Geometry check sheet. Reference: the model listing, model coordinates, mm. Face numbers are marked on the shaded views. A direction names the side the tool comes from. Round coordinates to 2 decimals unless told otherwise and drop trailing zeros. Write each loop counter-clockwise with the first axis right and the second up, starting at its lowest first coordinate (ties: lowest second). Pieces come first, ordered by that corner, then holes. Notation, with made-up numbers: (-21.5, 37.25) - (32.5, 37.25) arc R19 cw to (32.5, 70.25) - close; hole circle Ø1 at (75.5, 42). An arc over 180 degrees is marked (long way). Return JSON: item names as keys, results as strings.
```python
from build123d import *

# Parameters (mm, degrees)
SALIENTE_EXTRUIR1_DEPTH = 10
CROQUIS2_R              = 1.5
CORTAR_EXTRUIR1_DEPTH   = 10


with BuildPart() as part:
    # Croquis1 → Saliente-Extruir1 (new body)
    with BuildSketch(Plane.XY):
        Polygon((0, 0), (53, 0), (53, 25), (51, 25), (51, 27), (53, 27), (53, 29), (51, 29), (51, 31), (55, 31), (55, -2), (-2, -2), (-2, 31), (2, 31), (2, 29), (0, 29), (0, 27), (2, 27), (2, 25), (0, 25), align=None)
    extrude(amount=SALIENTE_EXTRUIR1_DEPTH)

    # Croquis2 → Cortar-Extruir1 (cut)
    with BuildSketch(Plane.XZ.offset(2)):
        with Locations((45, 5)):
            Circle(CROQUIS2_R)
        with Locations((8, 5)):
            Circle(CROQUIS2_R)
    extrude(amount=-CORTAR_EXTRUIR1_DEPTH, mode=Mode.SUBTRACT)


solid = part.part
```
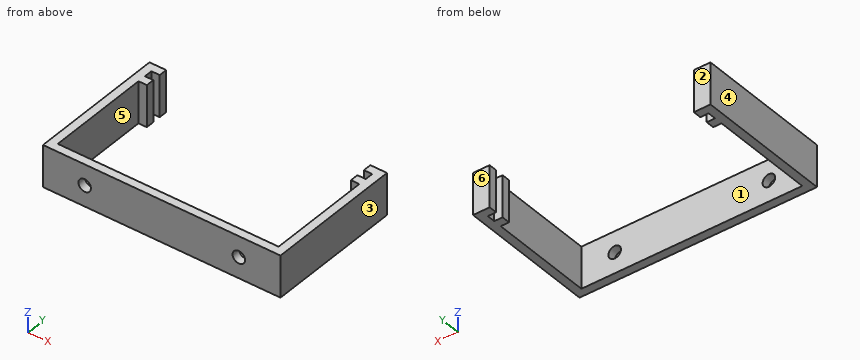
(1) Section check A-A, the plane x = 45. Enter the section's corners in (y, z), plus the area to 3 significant figures.
Response values:
{"outline": "(-2, 0) - (0, 0) - (0, 3.5) - (-2, 3.5) - close; (-2, 6.5) - (0, 6.5) - (0, 10) - (-2, 10) - close", "area": "14.0 mm^2"}
(2) Access from +Z, -Z, +X, -X, +Y, -Y to the whole of each face (thin tool, end or side, straight path). Record for the marked faces 5 and 6.
Response values:
{"face 5": "+Z, -Z", "face 6": "+Z, -Z, +X, -X, +Y"}
(3) Section check B-B, the plane y = 28. Enter the section's corners in (x, z), plus the area to 3 significant figures.
Response values:
{"outline": "(-2, 0) - (0, 0) - (0, 10) - (-2, 10) - close; (53, 0) - (55, 0) - (55, 10) - (53, 10) - close", "area": "40.0 mm^2"}
(4) Gauge pin test, flat end, axial feed: pin 1 (2 mm diameter, centred on x = 16, z = 3.5, fed in from +Y). Record the tip position at first contact, or that the pin passes through.
Response values:
{"pin 1": "stops at y = 0"}
(5) Material ranges on line 1 along X through (y, z) = (15, 8); line 2 along Z through (x, y) = (8, -1.05); line 3 along Y through (x, z) = (33.5, 5), recorded low to high. Write a range as [from, to].
Response values:
{"line 1": "x = [-2, 0], [53, 55]", "line 2": "z = [0, 3.5], [6.5, 10]", "line 3": "y = [-2, 0]"}
(6) Release check for a two-part mould opening along X. For the marked faces 1, 2, 3 and 4 record: pulls with the +X half, pulls with the -X half, needs draft (parallel to the pull), parting line crosses it, or undercut.
Response values:
{"face 1": "undercut", "face 2": "needs draft", "face 3": "pulls with the +X half", "face 4": "pulls with the -X half"}
(7) Section check C-C, the plane z = 5. Enter the section's corners in (x, y), plus the area to 3 significant figures.
Response values:
{"outline": "(-2, -2) - (6.5, -2) - (6.5, 0) - (0, 0) - (0, 25) - (2, 25) - (2, 27) - (0, 27) - (0, 29) - (2, 29) - (2, 31) - (-2, 31) - close; (9.5, -2) - (43.5, -2) - (43.5, 0) - (9.5, 0) - close; (46.5, -2) - (55, -2) - (55, 31) - (51, 31) - (51, 29) - (53, 29) - (53, 27) - (51, 27) - (51, 25) - (53, 25) - (53, 0) - (46.5, 0) - close", "area": "242 mm^2"}
(8) Section check D-D, the plane z = 1.25. Enter the section's corners in (x, y).
Response values:
{"outline": "(-2, -2) - (55, -2) - (55, 31) - (51, 31) - (51, 29) - (53, 29) - (53, 27) - (51, 27) - (51, 25) - (53, 25) - (53, 0) - (0, 0) - (0, 25) - (2, 25) - (2, 27) - (0, 27) - (0, 29) - (2, 29) - (2, 31) - (-2, 31) - close"}
